```python
from build123d import *

# Parameters (mm, degrees)
SKETCH074_R     = 2.5
SKETCH074_R_2   = 16
PAD042_DEPTH    = 15
SKETCH060_R     = 12.75
SKETCH060_R_2   = 12.5
PAD043_DEPTH    = 25
SKETCH064_R     = 60
POCKET036_DEPTH = 10.5


with BuildPart() as part:
    # Sketch074 → Pad042 (new body)
    with BuildSketch(Plane.XY):
        with BuildLine():
            ThreePointArc((-97.5, 110), (-106.338835, 106.338835), (-110, 97.5))
            Line((-110, 97.5), (-110, -97.5))
            ThreePointArc((-110, -97.5), (-106.338835, -106.338835), (-97.5, -110))
            Line((-97.5, -110), (97.5, -110))
            ThreePointArc((97.5, -110), (106.338835, -106.338835), (110, -97.5))
            Line((110, -97.5), (110, 97.5))
            ThreePointArc((110, 97.5), (106.338835, 106.338835), (97.5, 110))
            Line((97.5, 110), (-97.5, 110))
        make_face()
        with Locations((-97.5, 97.5)):
            Circle(SKETCH074_R, mode=Mode.SUBTRACT)
        with Locations((97.5, 97.5)):
            Circle(SKETCH074_R, mode=Mode.SUBTRACT)
        with Locations((-97.5, -97.5)):
            Circle(SKETCH074_R, mode=Mode.SUBTRACT)
        with Locations((97.5, -97.5)):
            Circle(SKETCH074_R, mode=Mode.SUBTRACT)
        Circle(SKETCH074_R_2, mode=Mode.SUBTRACT)
    extrude(amount=-PAD042_DEPTH)

    # Sketch060 → Pad043 (join)
    with BuildSketch(Plane(origin=(0, 0, 0), x_dir=(1, 0, 0), z_dir=(0, 0, -1))):
        with BuildLine():
            ThreePointArc((0, 18.75), (-18.75, 0), (0, -18.75))
            Line((0, -18.75), (100, -18.75))
            ThreePointArc((100, -18.75), (118.75, 0), (100, 18.75))
            Line((100, 18.75), (0, 18.75))
        make_face()
        Circle(SKETCH060_R, mode=Mode.SUBTRACT)
        with Locations((100, 0)):
            Circle(SKETCH060_R, mode=Mode.SUBTRACT)
        with Locations((50, 0)):
            Circle(SKETCH060_R_2, mode=Mode.SUBTRACT)
    extrude(amount=PAD043_DEPTH)

    # Sketch064 → Pocket036 (cut)
    with BuildSketch(Plane(origin=(0, 0, 0), x_dir=(1, 0, 0), z_dir=(0, 0, -1))):
        Circle(SKETCH064_R)
    extrude(amount=POCKET036_DEPTH, mode=Mode.SUBTRACT)


solid = part.part
```
Check sheet for the modelled part. Datum: model origin and axes. Units: mm. A direction names the side the tool comes from. Round coordinates to 2 decimals unless told otherwise and drop trailing zeros. Order: outer loops, then holes, each group sorted by start corner. A loop starts at its lowest first (then second) coordinate and runs counter-clockwise, first axis right, second up. Notation, with made-up numbers: (65, 28) -> (124, 28) arc R24 cw to (124, 49) -> close; hole circle Ø4 at (-12, 58). An arc over 180 degrees is marked (long way). One line per item, written item: value. Start each with the question number.
Q1. Cross-section at B-B (x = 43.5). Record the boundary of the cut face in (y, z), and give its area (3 significant figures).
Q2. Gauge pin test, flat ends, axial feed: pin 1 Ø3 at (x, z) = (27, -17.5) entering from -Y; pin 2 Ø8 at (y, z) = (12, -10) entering from +X; pin 3 Ø7 at (x, y) = (98.5, 0) entering from -Z. Record the tip position at first contact, or that the pin passes through.
Q3. Mould release check, pull along X, two halves, no side actions. Record for faces 1 (the face through (106.435, 106.241, -7.395)), 2 (the face through (-110, 1, -7)), 3 (the face through (110, 0, -7)): pulls with the +X half, pulls with the -X half, needs draft (parallel to the pull), parting line crosses it, or undercut.
Q4. Thickness scan on line 1 (X direction, y = -97, z = -5); line 2 (Y direction, x = -97.5, z = -3.75); line 3 (X direction, y = 0, z = -8). Record the ranges inside material, lowest first.
Q5. Cross-section at C-C (y = -56). Record the boundary of the cut face in (x, z).
Q6. Cross-section at A-A (y = 0). Record the boundary of the cut face in (x, z).
Q7. Set-up check for faces 4 (the face through (-18.745, -0.412, -19.93)), 5 (the face through (110, 56, -7)), 6 (the face through (-59.94, -2.64, -5.18)): record each of +Z, -Z, +X, -X, +Y, -Y from which the full face is reachable in a straight line by a thin tool's end or side.
Q8. Cross-section at D-D (x = -78). Record the boundary of the cut face in (y, z), and give its area (3 significant figures).
Completed:
1. outline: (-110, -15) -> (-18.75, -15) -> (-18.75, -25) -> (-10.68, -25) -> (-10.68, -15) -> (10.68, -15) -> (10.68, -25) -> (18.75, -25) -> (18.75, -15) -> (110, -15) -> (110, 0) -> (41.32, 0) -> (41.32, -10.5) -> (-41.32, -10.5) -> (-41.32, 0) -> (-110, 0) -> close
1. area: 2,590 mm²
2. pin 1: stops at y = -18.75
2. pin 2: stops at x = 116.96
2. pin 3: stops at z = -15
3. face 1: pulls with the +X half
3. face 2: pulls with the -X half
3. face 3: undercut
4. line 1: x = -110 to -99.95, -95.05 to 95.05, 99.95 to 110
4. line 2: y = -110 to -100, -95 to 95, 100 to 110
4. line 3: x = -110 to -60, 60 to 110, 112.75 to 118.75
5. outline: (-110, -15) -> (110, -15) -> (110, 0) -> (21.54, 0) -> (21.54, -10.5) -> (-21.54, -10.5) -> (-21.54, 0) -> (-110, 0) -> close
6. outline: (-110, -15) -> (-18.75, -15) -> (-18.75, -25) -> (-12.75, -25) -> (-12.75, -10.5) -> (-60, -10.5) -> (-60, 0) -> (-110, 0) -> close; (12.75, -25) -> (37.5, -25) -> (37.5, -15) -> (62.5, -15) -> (62.5, -25) -> (87.25, -25) -> (87.25, -15) -> (110, -15) -> (110, 0) -> (60, 0) -> (60, -10.5) -> (12.75, -10.5) -> close; (112.75, -25) -> (118.75, -25) -> (118.75, 0) -> (112.75, 0) -> close
7. face 4: -Z, -X
7. face 5: +Z, -Z, +X, +Y
7. face 6: +Z
8. outline: (-110, -15) -> (110, -15) -> (110, 0) -> (-110, 0) -> close
8. area: 3,300 mm²
